Could you check a few things on this model? Use its own coordinates, in mm. Coordinates: 2 decimals unless noted, no trailing zeros. Answer as a JSON object with one key per item and string values. Group by question number.
(1) Imagine slicing it at A-A, the plane y = -1.95. Give the number of separate pieces and of enclosed holes in the cut face, and give its area (3 significant figures).
(2) Will these pins go through, and if not, where does the flat tip stop? P1, Ø1, axis at y = -2.5, z = -2, coming from the -X side; P2, Ø4, axis at x = 33.78, z = -1.03, coming from the -Y side.
(3) Please list where these lines run through material, in increasing order: probe 1 along Z at (x, y) = (-51, -1.3); probe 2 along Z at (x, y) = (49, -0.15); probe 3 along Z at (x, y) = (-78.5, -2.1).
(4) We'd pull the mould along X, two halves only. Please class faces 1 (the cylindrical face through (36.088, -1.521, -1.988)), 2 (the flat face through (-33, -3, 0)): pulls with the +X half, pulls with the -X half, needs draft (parallel to the pull), parting line crosses it, or undercut.
from build123d import *

# Parameters (mm, degrees)
F2_DEPTH = 3
F1_R     = 2.5
F3_DEPTH = 3
F4_DEPTH = 3


with BuildPart() as f2:
    # F0 (on Front) → F2 (new body)
    with BuildSketch(Plane.XZ):
        with BuildLine():
            add(Edge.make_bspline(
                [(-96.9805282175, -0.8100506688), (-84.7869920978, 5.1468541776), (-43.2313518226, 10.3846705605), (26.8477938201, 4.0208678603), (73.1462007926, -1.0427900778)],
                knots=[0, 0, 0, 0, 0.374886421, 0.9004696716, 0.9004696716, 0.9004696716, 0.9004696716], degree=3))
            add(Edge.make_bspline(
                [(-97.5447368223, -7.1186651935), (-99.939251346, -6.5508492693), (-102.885147974, -5.168950634), (-100.0067471137, -2.3789404522), (-96.9805282175, -0.8100506688)],
                knots=[0.0564585679, 0.0564585679, 0.0564585679, 0.0564585679, 0.4847104148, 1, 1, 1, 1], degree=3))
            add(Edge.make_bspline(
                [(-96.5428845142, -7.3406707446), (-96.8949965543, -7.2673488468), (-97.22905608, -7.1935231869), (-97.5447368223, -7.1186651935)],
                knots=[0, 0, 0, 0, 0.0564585679, 0.0564585679, 0.0564585679, 0.0564585679], degree=3))
            add(Edge.make_bspline(
                [(-96.5428845142, -7.3406707446), (-80.7020161693, -9.4302402111), (-44.2471235075, -11.1181020976), (27.9226364637, -4.7767282079), (62.4434148738, -4.5021877215), (71.7967184236, -4.4503783305)],
                knots=[0, 0, 0, 0, 0.2987594418, 0.6837410955, 0.8381168975, 0.8381168975, 0.8381168975, 0.8381168975], degree=3))
            Line((71.7967184236, -4.4503783305), (72.2670713195, -3.2626866351))
            add(Edge.make_bspline(
                [(-97.3825784566, -6.0471531808), (-82.3468325761, -8.841713568), (-44.2551066449, -8.6286827794), (32.5707299039, -3.8332069517), (63.1103828262, -3.2710139005), (72.2670713195, -3.2626866351)],
                knots=[0, 0, 0, 0, 0.3131273629, 0.7122131732, 0.9019797674, 0.9019797674, 0.9019797674, 0.9019797674], degree=3))
            add(Edge.make_bspline(
                [(-97.3825784566, -6.0471531808), (-98.6588937786, -5.8946130057), (-100.1661659123, -5.1778479876), (-99.9138553768, -4.2244412327), (-99.8196757147, -4.047003109)],
                knots=[0, 0, 0, 0, 0.4440177242, 0.5425000514, 0.5425000514, 0.5425000514, 0.5425000514], degree=3))
            add(Edge.make_bspline(
                [(-99.8196757147, -4.047003109), (-99.3821638101, -3.2227137691), (-97.9006497107, -2.3042858417), (-96.3385477662, -1.6362179573)],
                knots=[0.5425000514, 0.5425000514, 0.5425000514, 0.5425000514, 1, 1, 1, 1], degree=3))
            add(Edge.make_bspline(
                [(-96.3385477662, -1.6362179573), (-85.7442874691, 3.2900694446), (-41.4192830911, 9.6956733525), (28.5693195485, 2.5855104747), (72.7689680214, -1.9953434339)],
                knots=[0, 0, 0, 0, 0.384923117, 0.9441251659, 0.9441251659, 0.9441251659, 0.9441251659], degree=3))
            Line((72.7689680214, -1.9953434339), (73.1462007926, -1.0427900778))
        make_face()
        with BuildLine():
            add(Edge.make_bspline(
                [(-96.5428845142, -7.3406707446), (-96.8949965543, -7.2673488468), (-97.22905608, -7.1935231869), (-97.5447368223, -7.1186651935)],
                knots=[0, 0, 0, 0, 0.0564585679, 0.0564585679, 0.0564585679, 0.0564585679], degree=3))
            ThreePointArc((-97.5447368223, -7.1186651935), (-97.052492706, -7.2688477084), (-96.5428845142, -7.3406707446))
        make_face()
        with BuildLine():
            Line((72.2670713195, -3.2626866351), (72.7689680214, -1.9953434339))
            add(Edge.make_bspline(
                [(-96.3385477662, -1.6362179573), (-85.7442874691, 3.2900694446), (-41.4192830911, 9.6956733525), (28.5693195485, 2.5855104747), (72.7689680214, -1.9953434339)],
                knots=[0, 0, 0, 0, 0.384923117, 0.9441251659, 0.9441251659, 0.9441251659, 0.9441251659], degree=3))
            add(Edge.make_bspline(
                [(-99.8196757147, -4.047003109), (-99.3821638101, -3.2227137691), (-97.9006497107, -2.3042858417), (-96.3385477662, -1.6362179573)],
                knots=[0.5425000514, 0.5425000514, 0.5425000514, 0.5425000514, 1, 1, 1, 1], degree=3))
            add(Edge.make_bspline(
                [(-97.3825784566, -6.0471531808), (-98.6588937786, -5.8946130057), (-100.1661659123, -5.1778479876), (-99.9138553768, -4.2244412327), (-99.8196757147, -4.047003109)],
                knots=[0, 0, 0, 0, 0.4440177242, 0.5425000514, 0.5425000514, 0.5425000514, 0.5425000514], degree=3))
            add(Edge.make_bspline(
                [(-97.3825784566, -6.0471531808), (-82.3468325761, -8.841713568), (-44.2551066449, -8.6286827794), (32.5707299039, -3.8332069517), (63.1103828262, -3.2710139005), (72.2670713195, -3.2626866351)],
                knots=[0, 0, 0, 0, 0.3131273629, 0.7122131732, 0.9019797674, 0.9019797674, 0.9019797674, 0.9019797674], degree=3))
        make_face()
    extrude(amount=F2_DEPTH)


with BuildPart() as f2b:
    # F1 (on Front) → F2, piece 2 (new body)
    with BuildSketch(Plane.XZ):
        with BuildLine():
            ThreePointArc((-45.542362095, -1.3708024857), (-51.4789804014, 2.1291274472), (-51.6671168627, -4.7598166753))
            Line((-51.6671168627, -4.7598166753), (-47.385046135, -4.7391830831))
            ThreePointArc((-47.385046135, -4.7391830831), (-46.0331411102, -3.2905337378), (-45.542362095, -1.3708024857))
        make_face()
        with BuildLine():
            Line((-47.385046135, -4.7391830831), (-51.6671168627, -4.7598166753))
            ThreePointArc((-51.6671168627, -4.7598166753), (-49.523087913, -5.3707560487), (-47.385046135, -4.7391830831))
        make_face()
    extrude(amount=F2_DEPTH)


with BuildPart() as f2c:
    # F1 (on Front) → F2, piece 3 (new body)
    with BuildSketch(Plane.XZ):
        with Locations((33.7789729238, -1.0305350879)):
            Circle(F1_R)
    extrude(amount=F2_DEPTH)


with BuildPart() as f3_tool:
    # F3 (cut): a face of the model
    f3_faces = [f2b.part.faces().sort_by_distance(p)[0] for p in [
        (-49.542362095, -3, -1.3708024857),
    ]]
    extrude(f3_faces, amount=-F3_DEPTH)


with BuildPart() as f2_1:
    add(f2.part)

    # F3: cut by f3_tool
    add(f3_tool.part, mode=Mode.SUBTRACT)


with BuildPart() as f2b_1:
    add(f2b.part)

    # F3: cut by f3_tool
    add(f3_tool.part, mode=Mode.SUBTRACT)


with BuildPart() as f4_tool:
    # F4 (cut): a face of the model
    f4_faces = [f2c.part.faces().sort_by_distance(p)[0] for p in [
        (33.7789729238, -3, -1.0305350879),
    ]]
    extrude(f4_faces, amount=-F4_DEPTH)


with BuildPart() as f2_2:
    add(f2_1.part)

    # F4: cut by f4_tool
    add(f4_tool.part, mode=Mode.SUBTRACT)


with BuildPart() as f2c_1:
    add(f2c.part)

    # F4: cut by f4_tool
    add(f4_tool.part, mode=Mode.SUBTRACT)


solid = f2_2.part
Result set:
{
 "1": {"separate pieces": "1", "enclosed holes": "2", "area": "1,980 mm^2"},
 "2": {"P1": "stops at x = -99.71", "P2": "passes through"},
 "3": {"probe 1": "z = -9.74 to -5.1, 2.35 to 7.4", "probe 2": "z = -4.75 to 1.51", "probe 3": "z = -9.12 to 4.91"},
 "4": {"face 1": "undercut", "face 2": "needs draft"}
}
